```python
from build123d import *

# Parameters (mm, degrees)
SKETCH_1_R          = 1.8000000000000025
SKETCH_1_R_2        = 1.8000000000000043
SKETCH_1_R_3        = 1.8000000000000005
SKETCH_1_R_4        = 1.8000000000000007
EXTRUDE_1_DEPTH     = 42
SKETCH_2_R          = 6.000000000000001
CUT_EXTRUDE_1_DEPTH = 58.404268133998535
SKETCH_3_R          = 6.000000000000002
CUT_EXTRUDE_2_DEPTH = 58.404268133998535
SKETCH_5_W          = 12
SKETCH_5_H          = 15.000000000000005
SKETCH_5_H_2        = 15.000000000000002
CUT_EXTRUDE_3_DEPTH = 58.404268133998535
EXTRUDE_2_DEPTH     = 2.1
EXTRUDE_3_DEPTH     = 1
EXTRUDE_START       = 2.1
EXTRUDE_4_DEPTH     = 2.1
EXTRUDE_START_2     = 1
EXTRUDE_5_DEPTH     = 1


with BuildPart() as part:
    # 草图1 → 凸台-拉伸1 (new body)
    with BuildSketch(Plane(origin=(0, 0, 0), x_dir=(-1, 0, 0), z_dir=(0, 0, 1))):
        with BuildLine():
            Line((-17.499999999999996, 15), (-17.499999999999996, -15.000000000000007))
            ThreePointArc((-17.499999999999996, -15.000000000000007), (-16.767766952966365, -16.767766952966372), (-15, -17.500000000000007))
            Line((-15, -17.500000000000007), (15.000000000000004, -17.500000000000007))
            ThreePointArc((15.000000000000004, -17.500000000000007), (16.76776695296637, -16.767766952966376), (17.5, -15.00000000000001))
            Line((17.5, -15.00000000000001), (17.5, 14.999999999999996))
            ThreePointArc((17.5, 14.999999999999996), (16.76776695296637, 16.76776695296636), (15.000000000000004, 17.499999999999996))
            Line((15.000000000000004, 17.499999999999996), (-15, 17.499999999999996))
            ThreePointArc((-15, 17.499999999999996), (-16.767766952966365, 16.767766952966365), (-17.499999999999996, 15))
        make_face()
        with Locations((-15.000000000000004, -15.00000000000001)):
            Circle(SKETCH_1_R, mode=Mode.SUBTRACT)
        with Locations((15.000000000000004, -15.00000000000001)):
            Circle(SKETCH_1_R_2, mode=Mode.SUBTRACT)
        with Locations((15.000000000000004, 14.999999999999996)):
            Circle(SKETCH_1_R_3, mode=Mode.SUBTRACT)
        with Locations((-15, 15)):
            Circle(SKETCH_1_R_4, mode=Mode.SUBTRACT)
        with BuildLine():
            Line((15.604722413530899, -11.417049414734192), (15.604722413530899, 11.41704941481964))
            ThreePointArc((15.604722413530899, 11.41704941481964), (15.349600753639777, 12.084241863325458), (14.714404940145743, 12.41098197902667))
            ThreePointArc((14.714404940145743, 12.41098197902667), (13.158183898644735, 13.15818233801838), (12.410982220986185, 14.714402746377065))
            ThreePointArc((12.410982220986185, 14.714402746377065), (12.084242685294747, 15.349600017363324), (11.417049414775391, 15.604722413530212))
            Line((11.417049414775391, 15.604722413530212), (-11.417049414778536, 15.604722413530212))
            ThreePointArc((-11.417049414778536, 15.604722413530212), (-12.084241863278942, 15.349600753643644), (-12.410981978984013, 14.714404940159108))
            ThreePointArc((-12.410981978984013, 14.714404940159108), (-13.158182337972896, 13.158183898648431), (-14.714402746337697, 12.41098222098531))
            ThreePointArc((-14.714402746337697, 12.41098222098531), (-15.34960001732269, 12.084242685293246), (-15.604722413489107, 11.41704941477461))
            Line((-15.604722413489107, 11.41704941477461), (-15.604722413489107, -11.417049414779225))
            ThreePointArc((-15.604722413489107, -11.417049414779225), (-15.349600753597985, -12.084241863285039), (-14.714404940103952, -12.410981978986248))
            ThreePointArc((-14.714404940103952, -12.410981978986248), (-13.158183898602942, -13.158182337977962), (-12.410982220944396, -14.714402746336651))
            ThreePointArc((-12.410982220944396, -14.714402746336651), (-12.084242685252958, -15.34960001732291), (-11.417049414733604, -15.604722413489796))
            Line((-11.417049414733604, -15.604722413489796), (11.417049414820326, -15.604722413489796))
            ThreePointArc((11.417049414820326, -15.604722413489796), (12.084241863320731, -15.349600753603227), (12.410981979025802, -14.714404940118692))
            ThreePointArc((12.410981979025802, -14.714404940118692), (13.158182338014687, -13.158183898608014), (14.71440274637949, -12.410982220944893))
            ThreePointArc((14.71440274637949, -12.410982220944893), (15.34960001736448, -12.084242685252828), (15.604722413530899, -11.417049414734192))
        make_face(mode=Mode.SUBTRACT)
    extrude(amount=EXTRUDE_1_DEPTH)

    # 草图2 → 切除-拉伸1 (cut, through all)
    with BuildSketch(Plane(origin=(0, 17.500000000000007, 0), x_dir=(1, 0, 0), z_dir=(0, 1, 0))):
        with Locations(Location((0, -11.999999999999998, 0), (0, 0, 270))):
            Circle(SKETCH_2_R)
    extrude(amount=-CUT_EXTRUDE_1_DEPTH, mode=Mode.SUBTRACT)

    # 草图3 → 切除-拉伸2 (cut, through all)
    with BuildSketch(Plane.ZY.offset(17.5)):
        with Locations((30, 0)):
            Circle(SKETCH_3_R)
    extrude(amount=-CUT_EXTRUDE_2_DEPTH, mode=Mode.SUBTRACT)

    # 草图5 → 切除-拉伸3 (cut, through all)
    with BuildSketch(Plane(origin=(17.499999999999996, 0, 0), x_dir=(0, 0, -1), z_dir=(1, 0, 0))):
        Polygon((-30, -24.974265818952347), (-30, -15), (-42, -15), (-42, 15.000000000000007), (-30, 15.000000000000007), (-30, 23.87950348168345), (-47.41212790980853, 25.238249525472156), (-47.41212790980853, -24.974265818952347), align=None)
        with BuildLine():
            Line((-42, -15), (-30, -15))
            Line((-30, -15), (-30, -6.000000000000003))
            ThreePointArc((-29.999999999999925, -6.000000000000003), (-36, -1.93e-15), (-29.999999999999932, 6.000000000000003))
            Line((-30, 6.000000000000003), (-30, 15.000000000000007))
            Line((-30, 15.000000000000007), (-42, 15.000000000000007))
            Line((-42, 15.000000000000007), (-42, -15))
        make_face()
        with Locations((-6, 7.500000000000003)):
            Rectangle(SKETCH_5_W, SKETCH_5_H)
        Polygon((0, 15.000000000000007), (0, 0), (0, -15), (-12, -15), (-12, -24.974265818952347), (12.116605042765016, -24.974265818952347), (12.116605042765016, 23.87950348168345), (-12, 23.87950348168345), (-12, 15.000000000000007), align=None)
        with Locations((-6, -7.500000000000001)):
            Rectangle(SKETCH_5_W, SKETCH_5_H_2)
    extrude(amount=-CUT_EXTRUDE_3_DEPTH, mode=Mode.SUBTRACT)

    # 草图6 → 凸台-拉伸2 (add)
    with BuildSketch(Plane(origin=(0, 15.604722413489796, 0), x_dir=(-1, 0, 0), z_dir=(0, -1, 0))):
        with BuildLine():
            Line((-6.000000000000001, -11.999999999999998), (-6.500000000000001, -11.999999999999998))
            ThreePointArc((-6.500000000000001, -11.999999999999998), (-1.19e-15, -18.5), (6.500000000000001, -11.999999999999998))
            Line((6.500000000000001, -11.999999999999998), (6.000000000000001, -11.999999999999998))
            ThreePointArc((6.000000000000001, -11.999999999999998), (-1.1e-15, -18), (-6.000000000000001, -11.999999999999998))
        make_face()
    extrude_2 = extrude(amount=EXTRUDE_2_DEPTH)

    # 草图7 → 凸台-拉伸3 (add)
    with BuildSketch(Plane(origin=(0, 13.504722413489795, 0), x_dir=(-1, 0, 0), z_dir=(0, -1, 0))):
        with BuildLine():
            Line((-6.500000000000002, -11.999999999999998), (-5.750000000000001, -11.999999999999998))
            ThreePointArc((-5.750000000000001, -11.999999999999998), (-1.06e-15, -17.75), (5.750000000000001, -11.999999999999998))
            Line((5.750000000000001, -11.999999999999998), (6.500000000000002, -11.999999999999998))
            ThreePointArc((6.500000000000002, -11.999999999999998), (-1.19e-15, -18.5), (-6.500000000000002, -11.999999999999998))
        make_face()
    extrude_3 = extrude(amount=EXTRUDE_3_DEPTH)

    # 镜向1: 凸台-拉伸2, 凸台-拉伸3 across plane
    add(extrude_2.mirror(Plane(origin=(0, 0, 0), x_dir=(0, 0, 1), z_dir=(0, -1, 0))))
    add(extrude_3.mirror(Plane(origin=(0, 0, 0), x_dir=(0, 0, 1), z_dir=(0, -1, 0))))

    # 草图8 → 凸台-拉伸4 (add)
    with BuildSketch(Plane.ZY.offset(-15.604722413489107).offset(EXTRUDE_START)):
        with BuildLine():
            Line((30, -6.500000000000001), (30, -6.000000000000003))
            ThreePointArc((30, -6.000000000000003), (23.999999999999996, 7.3e-16), (30, 6.000000000000003))
            Line((30, 6.000000000000003), (30, 6.500000000000001))
            ThreePointArc((30, 6.500000000000001), (23.5, 8e-16), (30, -6.500000000000001))
        make_face()
    extrude_4 = extrude(amount=-EXTRUDE_4_DEPTH)

    # 草图9 → 凸台-拉伸5 (add)
    with BuildSketch(Plane.ZY.offset(-13.504722413489107).offset(EXTRUDE_START_2)):
        with BuildLine():
            Line((30, -6.500000000000001), (30, -5.750000000000003))
            ThreePointArc((30, -5.750000000000003), (24.249999999999996, 7e-16), (30, 5.750000000000003))
            Line((30, 5.750000000000003), (30, 6.500000000000001))
            ThreePointArc((30, 6.500000000000001), (23.5, 8e-16), (30, -6.500000000000001))
        make_face()
    extrude_5 = extrude(amount=-EXTRUDE_5_DEPTH)

    # 镜向2: 凸台-拉伸4, 凸台-拉伸5 across plane
    add(extrude_4.mirror(Plane.ZY))
    add(extrude_5.mirror(Plane.ZY))


solid = part.part
```
The model under review builds one solid part; all positions refer to its coordinate system, in mm. A direction names the side the tool comes from. Give positions to 0.01 mm unless a question says otherwise; leave off trailing zeros. Write each loop counter-clockwise with the first axis right and the second up, starting at its lowest first coordinate (ties: lowest second). Pieces come first, ordered by that corner, then holes. Notation, with made-up numbers: (-11, -24) -> (4, -24) arc R13 ccw to (4, -8) -> close; hole circle Ø7 at (58, 84). An arc over 180 degrees is marked (long way). Put each result on its own line as item: value.
(1) We need section A-A, the plane y = -7. Give the boundary of the cut face in (x, z), and give its area (3 significant figures).
Results are:
outline: (-17.5, 12) -> (-15.6, 12) -> (-15.6, 30) -> (-17.5, 30) -> close; (15.6, 12) -> (17.5, 12) -> (17.5, 30) -> (15.6, 30) -> close
area: 68.2 mm²
(2) We need section D-D, the plane y = 14. Give the boundary of the cut face in (x, z).
Results are:
outline: (-17.5, 12) -> (-16.5, 12) -> (-16.5, 30) -> (-17.5, 30) -> close; (-13.5, 12) -> (-12.59, 12) -> (-12.59, 30) -> (-13.5, 30) -> close; (-6.5, 12) -> (-6, 12) arc R6 cw to (6, 12) -> (6.5, 12) arc R6.5 ccw to start; (12.59, 12) -> (13.5, 12) -> (13.5, 30) -> (12.59, 30) -> close; (16.5, 12) -> (17.5, 12) -> (17.5, 30) -> (16.5, 30) -> close
(3) For pin 1 Ø2 at (x, z) = (2, 14) entering from +Y; pin 2 Ø1 at (x, z) = (4.5, 15) entering from +Y, all flat-tipped, find the tip position at first contact; note any pin that passes through.
Results are:
pin 1: through
pin 2: y = 13.5
(4) We need section C-C, the plane z = 20.5. Give the boundary of the cut face in (x, y).
Results are:
outline: (-17.5, -15) arc R2.5 ccw to (-15, -17.5) -> (15, -17.5) arc R2.5 ccw to (17.5, -15) -> (17.5, 15) arc R2.5 ccw to (15, 17.5) -> (-15, 17.5) arc R2.5 ccw to (-17.5, 15) -> close; hole circle Ø3.6 at (-15, -15); hole circle Ø3.6 at (-15, 15); hole (-15.6, -11.42) arc R1 ccw to (-14.71, -12.41) arc R2.6 cw to (-12.41, -14.71) arc R1 ccw to (-11.42, -15.6) -> (11.42, -15.6) arc R1 ccw to (12.41, -14.71) arc R2.6 cw to (14.71, -12.41) arc R1 ccw to (15.6, -11.42) -> (15.6, 11.42) arc R1 ccw to (14.71, 12.41) arc R2.6 cw to (12.41, 14.71) arc R1 ccw to (11.42, 15.6) -> (-11.42, 15.6) arc R1 ccw to (-12.41, 14.71) arc R2.6 cw to (-14.71, 12.41) arc R1 ccw to (-15.6, 11.42) -> close; hole circle Ø3.6 at (15, -15); hole circle Ø3.6 at (15, 15)
(5) We need section B-B, the plane x = 0. Give the boundary of the cut face in (y, z).
Results are:
outline: (-17.5, 18) -> (-13.5, 18) -> (-13.5, 17.75) -> (-12.5, 17.75) -> (-12.5, 18.5) -> (-15.6, 18.5) -> (-15.6, 30) -> (-17.5, 30) -> close; (12.5, 17.75) -> (13.5, 17.75) -> (13.5, 18) -> (17.5, 18) -> (17.5, 30) -> (15.6, 30) -> (15.6, 18.5) -> (12.5, 18.5) -> close
(6) The part is to be moulded in two halves that separate along X. For faces 1 (the flat face through (0, -12.505, 18)), 2 (the flat face through (-17.5, 0, 21)), 3 (the flat face through (17.5, 0, 21)), 4 (the cylindrical face through (-0.1, -14.1, 18.5)), say which applies: pulls with the +X half, pulls with the -X half, needs draft (parallel to the pull), parting line crosses it, or undercut.
Results are:
face 1: undercut
face 2: pulls with the -X half
face 3: pulls with the +X half
face 4: undercut
(7) Tool access review of faces 5 (the flat face through (16, -3, 12)), 6 (the cylindrical face through (14, 0.1, 23.5)), 7 (the cylindrical face through (13.176, 13.141, 20.874)): name each direction out of +Z, -Z, +X, -X, +Y, -Y from which nothing blocks a thin tool from reaching the whole face with its end or side.
Results are:
face 5: -Z, +X, -X, +Y, -Y
face 6: -Z
face 7: +Z, -Z
(8) To check wall thickness, follow probe 1 along X at (y, z) = (6.5, 22.5); probe 2 along Y at (x, z) = (15, 21.5); probe 3 along Y at (x, z) = (15, 25). State the ranges of each line that lie inside material, in increasing order. Write a range as from..to.
Results are:
probe 1: -17.5..-15.6, 15.6..17.5
probe 2: -17.5..-16.8, -13.2..-12.34, 12.34..13.2, 16.8..17.5
probe 3: -17.5..-16.8, -13.2..-12.34, -4.15..-3.32, 3.32..4.15, 12.34..13.2, 16.8..17.5
